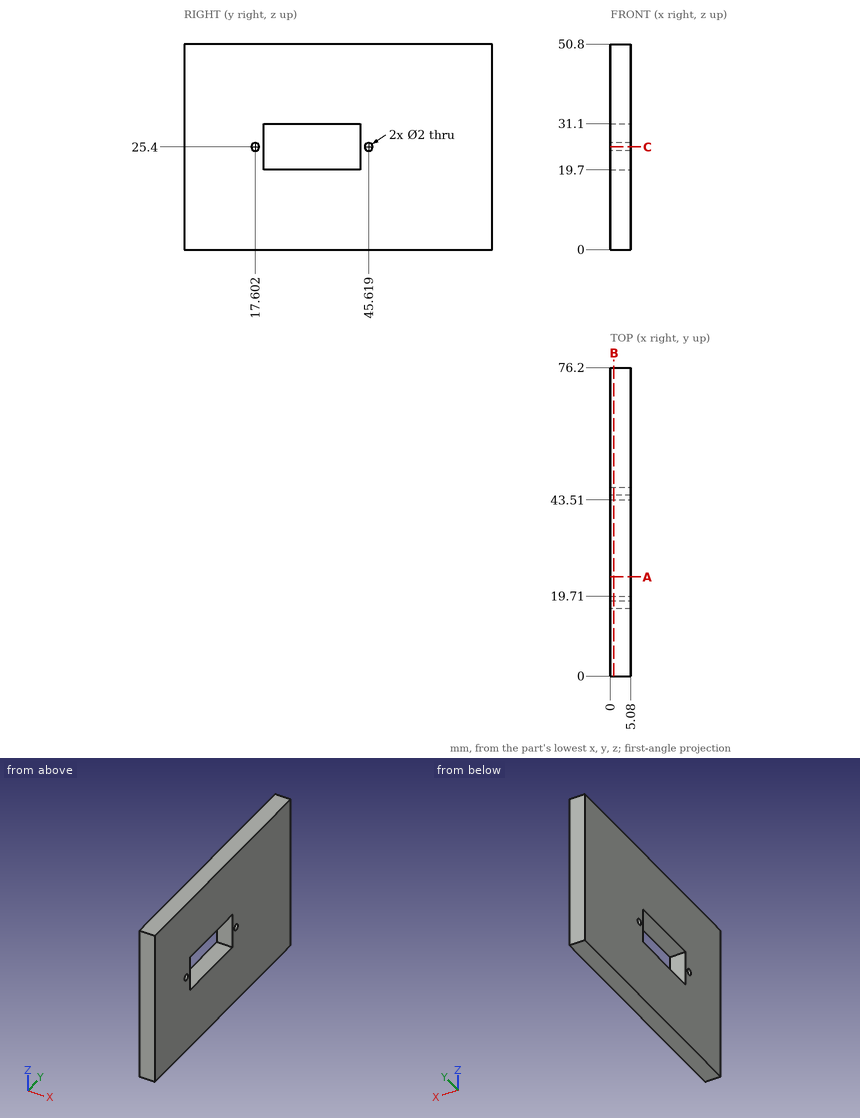
Geometry: see drawing. Coordinates: mm, zero at the bounding-box minimum. Coordinates: 2 decimals unless noted, no trailing zeros. Order: outer loops, then holes, each group sorted by start corner. A loop starts at its lowest first (then second) coordinate and runs counter-clockwise, first axis right, second up. Notation, with made-up numbers: (69, 37) -> (89, 37) arc R18 cw to (89, 45) -> close; hole circle Ø7 at (45, 71.25). An arc over 180 degrees is marked (long way). Write each question's results on one line, items separated by ' | '. Start each with the question number.
1) Material intervals for line 1 along Y through (x, z) = (2.3, 27.5); line 2 along Z through (x, y) = (4.8, 42); line 3 along Z through (x, y) = (4.75, 45) (1 decimal), sorted ascending.
2) Cut plane B-B, the plane x = 0.85. Output: boundary loops of the cut face in (y, z).
3) Cut plane C-C, the plane z = 25.4. Output: boundary loops of the cut face in (x, y), and give its area (3 significant figures).
4) Cut plane A-A, the plane y = 24.5. Output: boundary loops of the cut face in (x, z).
Checks:
1) line 1: 0 to 19.71, 43.51 to 76.2 | line 2: 0 to 19.7, 31.1 to 50.8 | line 3: 0 to 24.6, 26.2 to 50.8
2) outline: (0, 0) -> (76.2, 0) -> (76.2, 50.8) -> (0, 50.8) -> close; hole circle Ø2 at (17.6, 25.4); hole (19.71, 19.7) -> (43.51, 19.7) -> (43.51, 31.1) -> (19.71, 31.1) -> close; hole circle Ø2 at (45.62, 25.4)
3) outline: (0, 0) -> (5.08, 0) -> (5.08, 16.6) -> (0, 16.6) -> close; (0, 18.6) -> (5.08, 18.6) -> (5.08, 19.71) -> (0, 19.71) -> close; (0, 43.51) -> (5.08, 43.51) -> (5.08, 44.62) -> (0, 44.62) -> close; (0, 46.62) -> (5.08, 46.62) -> (5.08, 76.2) -> (0, 76.2) -> close | area: 246 mm^2
4) outline: (0, 0) -> (5.08, 0) -> (5.08, 19.7) -> (0, 19.7) -> close; (0, 31.1) -> (5.08, 31.1) -> (5.08, 50.8) -> (0, 50.8) -> close
